Here's how the part is built. I have some questions about the finished solid (model axes, mm). Face numbers are marked on the shaded views. A direction names the side the tool comes from. Round coordinates to 2 decimals unless told otherwise and drop trailing zeros. Write each loop counter-clockwise with the first axis right and the second up, starting at its lowest first coordinate (ties: lowest second). Pieces come first, ordered by that corner, then holes. Notation, with made-up numbers: (89, -4.75) -> (107, -4.75) arc R11 ccw to (107, 4.25) -> close; hole circle Ø10 at (68.5, -23). An arc over 180 degrees is marked (long way). Answer in a Markdown table with one row per item. Add a question column.
from build123d import *

# Parameters (mm, degrees)
BOSS_EXTRUDE1_DEPTH = 13.5
SKETCH2_W           = 10
SKETCH2_H           = 1.5
CUT_EXTRUDE1_DEPTH  = 27
SKETCH3_R           = 1
CUT_EXTRUDE2_DEPTH  = 3.6
SKETCH4_W           = 6
SKETCH4_H           = 2
BOSS_EXTRUDE2_DEPTH = 3
SKETCH5_R           = 1.5
CUT_EXTRUDE3_DEPTH  = 9
BOSS_EXTRUDE3_DEPTH = 2
SKETCH8_W           = 6
SKETCH8_H           = 3
CUT_EXTRUDE4_DEPTH  = 10


with BuildPart() as part:
    # Sketch1 → Boss-Extrude1 (new, symmetric)
    with BuildSketch(Plane.XY):
        Polygon((0, 11), (0, 0), (6, 0), (6, 2), (2, 2), (2, 11), align=None)
    extrude(amount=BOSS_EXTRUDE1_DEPTH, both=True)

    # Sketch2 → Cut-Extrude1 (cut)
    with BuildSketch(Plane(origin=(2, 0, 0), x_dir=(0, 0, -1), z_dir=(1, 0, 0))):
        with Locations((-8.5, 10.25)):
            Rectangle(SKETCH2_W, SKETCH2_H)
    extrude(amount=-CUT_EXTRUDE1_DEPTH, mode=Mode.SUBTRACT)

    # Sketch3 → Cut-Extrude2 (cut)
    with BuildSketch(Plane.ZY):
        with Locations(Location((-11.75, 9.25, 0), (0, 0, 270))):
            Circle(SKETCH3_R)
        with Locations(Location((11.723777669, 1.75, 0), (0, 0, 270))):
            Circle(SKETCH3_R)
    extrude(amount=-CUT_EXTRUDE2_DEPTH, mode=Mode.SUBTRACT)

    # Sketch4 → Boss-Extrude2 (add)
    with BuildSketch(Plane.XY.offset(13.5)):
        with Locations((3, 1)):
            Rectangle(SKETCH4_W, SKETCH4_H)
    extrude(amount=BOSS_EXTRUDE2_DEPTH)

    # Sketch5 → Cut-Extrude3 (cut)
    with BuildSketch(Plane(origin=(0, 2, 0), x_dir=(1, 0, 0), z_dir=(0, 1, 0))):
        with Locations(Location((4, 4.7, 0), (0, 0, 180))):
            Circle(SKETCH5_R)
        with Locations(Location((4, -4.7, 0), (0, 0, 270))):
            Circle(SKETCH5_R)
    extrude(amount=-CUT_EXTRUDE3_DEPTH, mode=Mode.SUBTRACT)

    # Sketch7 → Boss-Extrude3 (add)
    with BuildSketch(Plane.XY):
        Polygon((2, 8.5), (6, 2), (2, 2), align=None)
    extrude(amount=BOSS_EXTRUDE3_DEPTH)

    # Sketch8 → Cut-Extrude4 (cut)
    with BuildSketch(Plane(origin=(0, 2, 0), x_dir=(1, 0, 0), z_dir=(0, 1, 0))):
        with Locations((3, -15)):
            Rectangle(SKETCH8_W, SKETCH8_H)
    extrude(amount=-CUT_EXTRUDE4_DEPTH, mode=Mode.SUBTRACT)


solid = part.part
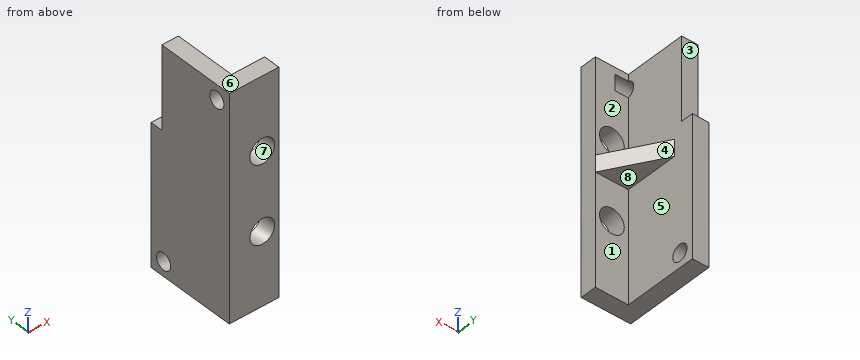
Item 1: If we section it at D-D on z = 9.5: Please give me the cut outline in (x, y).
Item 2: On a 3-axis mill with a long thin cutter (end or side, diameter ignored), from which of +Z, -Z, +X, -X, +Y, -Y can I reach the whole of each face in a straight line? I mean the marked faces 1, 2, 3 and 4. Say none if no direction works.
Item 3: I need wall thicknesses on line 1 along Z through (x, y) = (0.5, 1.75); line 2 along Z through (x, y) = (1.6, 9.25); line 3 along X through (y, z) = (0.75, 4.7). Which ranges of each line are inside material? Lowest first, please. Write a range as from..to.
Item 4: If we section it at B-B on y = 1.75: Please give me the cut outline in (x, z).
Item 5: If we section it at A-A on x = 4: Please give me the cut outline in (y, z).
Item 6: If we mould it in two halves opening along Z, with no side actions, what happens to the marked faces 5, 6, 7 and 8? For each: pulls with the +Z half, pulls with the -Z half, needs draft (parallel to the pull), parting line crosses it, or undercut.
Item 7: If we section it at C-C on z = -11.75: Please give me the cut outline in (x, y), then the cut area to 3 significant figures.
Item 8: For P1, Ø2.5, axis at y = 9.25, z = -11.75, coming from the +X side; P2, Ø1, axis at x = 4.5, y = 5.5, coming from the +Z side; P3, Ø0.6, axis at x = 1.5, z = 7.5, coming from the +Y side; P4, Ø1.6, axis at y = 1.75, z = 11.72, coming from the -X side, each with a flat end and sliding along its axis, tell me the tip position at first contact or that it passes through.
Results list:
| question | item | result |
|---|---|---|
| 1 | outline | (0, 0) -> (6, 0) -> (6, 2) -> (2, 2) -> (2, 9.5) -> (0, 9.5) -> close |
| 2 | face 1 | -Z, +X, +Y |
| 2 | face 2 | +Z, +X, +Y |
| 2 | face 3 | +Z, +X, -X, +Y |
| 2 | face 4 | +Z, -Z, +X, +Y |
| 3 | line 1 | -13.5..10.72, 12.72..13.5 |
| 3 | line 2 | -13.5..-12.75, -10.75..13.5 |
| 3 | line 3 | 0..2.5, 5.5..6 |
| 4 | outline | (0, -13.5) -> (6, -13.5) -> (6, 13.5) -> (0, 13.5) -> (0, 12.72) -> (3.6, 12.72) -> (3.6, 10.72) -> (0, 10.72) -> close; hole circle Ø3 at (4, -4.7); hole circle Ø3 at (4, 4.7) |
| 5 | outline | (0, -13.5) -> (2, -13.5) -> (2, -6.2) -> (0, -6.2) -> close; (0, -3.2) -> (2, -3.2) -> (2, 0) -> (5.25, 0) -> (5.25, 2) -> (2, 2) -> (2, 3.2) -> (0, 3.2) -> close; (0, 6.2) -> (2, 6.2) -> (2, 13.5) -> (0, 13.5) -> close |
| 6 | face 5 | needs draft |
| 6 | face 6 | pulls with the +Z half |
| 6 | face 7 | undercut |
| 6 | face 8 | pulls with the -Z half |
| 7 | outline | (0, 0) -> (6, 0) -> (6, 2) -> (2, 2) -> (2, 8.25) -> (0, 8.25) -> close; (0, 10.25) -> (2, 10.25) -> (2, 11) -> (0, 11) -> close |
| 7 | area | 26.0 mm² |
| 8 | P1 | x = 2 |
| 8 | P2 | through |
| 8 | P3 | y = 9.5 |
| 8 | P4 | x = 3.6 |
